Build history of the part. All positions in model axes, mm. A direction names the side the tool comes from. Give positions to 0.01 mm unless a question says otherwise; leave off trailing zeros. Loops run counter-clockwise (first coordinate to the right, second up) from the corner with the lowest first, then second, coordinate; pieces in that order, holes last. Notation, with made-up numbers: (-25.75, 66) -> (28.25, 66) arc R22 cw to (28.25, 98) -> close; hole circle Ø2 at (1, -25.75). An arc over 180 degrees is marked (long way). One line per question, with ' | ' between items. Start each with the question number.
(1) Flat gauge pins, fed straight in: pin 1 Ø12 at (x, y) = (3, 116) entering from +Z; pin 2 Ø9 at (x, y) = (7, 243) entering from -Z; pin 3 Ø4 at (x, z) = (7.5, 74) entering from -Y. Where does each tip first touch, or does it go through?
(2) Drill centre lines: L1, parallel to Y at x = 4, z = -6.5; L2, parallel to Z at x = -9.5, y = 295; L3, parallel to Z at x = 0.5, y = 117.5. Where is each one in solid material? Low to high. Write a range as from..to.
(3) Slice it at A-A, the plane z = -11. Write the cut outline in (x, y).
(4) Slice it at B-B, the plane x = 13.5. Write the cut outline in (y, z), then the cut area to 3 significant figures.
(5) Slice it at D-D, the plane x = -8.5. Write the cut outline in (y, z).
(6) Slice it at C-C, the plane y = 157.5. Write the cut outline in (x, z), then the cut area to 3 significant figures.
(7) 3-axis set-ups, long thin cutter, end or side, ignore diameter. For faces 1 (the face through (25.865, 113.39, 10.724)), 2 (the face through (22, 230, 21)), 3 (the face through (0, 245, -28)), 4 (the face through (0, 244, 28)): which of +Z, -Z, +X, -X, +Y, -Y reach the whole face in a straight line?
```python
from build123d import *

# Parameters (mm, degrees)
SKETCH1_R           = 28
BOSS_EXTRUDE1_DEPTH = 230
BOSS_EXTRUDE2_DEPTH = 28


with BuildPart() as part:
    # Sketch1 → Boss-Extrude1 (new body)
    with BuildSketch(Plane(origin=(0, 0, 0), x_dir=(1, 0, 0), z_dir=(0, 1, 0))):
        Circle(SKETCH1_R)
    extrude(amount=BOSS_EXTRUDE1_DEPTH)

    # Sketch2 → Boss-Extrude2 (add, symmetric)
    with BuildSketch(Plane(origin=(0, 0, 0), x_dir=(0, 0, -1), z_dir=(1, 0, 0))):
        with BuildLine():
            Line((6.592878428, 292.481093562), (95, 370))
            Line((95, 370), (120, 370))
            Line((120, 370), (120, 340))
            Line((120, 340), (28, 259.330713798))
            Line((28, 259.330713798), (28, 230))
            Line((28, 230), (-28, 230))
            Line((-28, 230), (-28, 259.330713798))
            Line((-28, 259.330713798), (-120, 340))
            Line((-120, 340), (-120, 370))
            Line((-120, 370), (-95, 370))
            Line((-95, 370), (-6.592878428, 292.481093562))
            ThreePointArc((-6.592878428, 292.481093562), (0, 290), (6.592878428, 292.481093562))
        make_face()
    extrude(amount=BOSS_EXTRUDE2_DEPTH, both=True)


solid = part.part
```
Final values:
1) pin 1: z = 28 | pin 2: z = -28 | pin 3: y = 297.91
2) L1: 0..292.4 | L2: -68.68..-9.47, 9.47..68.68 | L3: -28..28
3) outline: (-28, 230) -> (-25.75, 230) -> (-25.75, 0) -> (25.75, 0) -> (25.75, 230) -> (28, 230) -> (28, 296.35) -> (-28, 296.35) -> close
4) outline: (0, -24.53) -> (230, -24.53) -> (230, -28) -> (259.33, -28) -> (340, -120) -> (370, -120) -> (370, -95) -> (292.48, -6.59) arc R10 cw to (292.48, 6.59) -> (370, 95) -> (370, 120) -> (340, 120) -> (259.33, 28) -> (230, 28) -> (230, 24.53) -> (0, 24.53) -> close | area: 24,200 mm2
5) outline: (0, -26.68) -> (230, -26.68) -> (230, -28) -> (259.33, -28) -> (340, -120) -> (370, -120) -> (370, -95) -> (292.48, -6.59) arc R10 cw to (292.48, 6.59) -> (370, 95) -> (370, 120) -> (340, 120) -> (259.33, 28) -> (230, 28) -> (230, 26.68) -> (0, 26.68) -> close
6) outline: circle Ø56 at (0, 0) | area: 2,460 mm2
7) face 1: -Y | face 2: +Z, +X, -Y | face 3: -Z, +X, -X, -Y | face 4: +Z, +X, -X, -Y
